Verification items for the finished model (mm, model axes). A direction names the side the tool comes from. Give positions to 0.01 mm unless a question says otherwise; leave off trailing zeros. Order: outer loops, then holes, each group sorted by start corner. A loop starts at its lowest first (then second) coordinate and runs counter-clockwise, first axis right, second up. Notation, with made-up numbers: (13.25, 89) - (67.25, 89) arc R13 cw to (67.25, 99) - close; hole circle Ø8 at (64.25, 20.5). An arc over 180 degrees is marked (long way). Answer as a JSON object with one key per item and string values. Group by question number.
(1) Section check C-C (z = -22). Record the boundary of the cut face in (x, y).
(2) Section check A-A (x = -1.5). Count the separate pieces of the cut face and the enclosed holes in it, then the cut area to 3 significant figures.
(3) Depth check by flat-ended pin: pin 1 Ø1.9 at (x, z) = (-21.5, -22) entering from +Y; pin 2 Ø0.6 at (x, y) = (-15, 6) entering from -Z. Enter the tip coordinate at first touch or a pass-through.
(4) Section check B-B (z = -7.75). Record the boundary of the cut face in (x, y).
(5) Access from +Z, -Z, +X, -X, +Y, -Y to the whole of each face (thin tool, end or side, straight path). Record for faces 1 (the face through (-11, 6.5, -2)), 2 (the face through (-11, 4, -20.5)), 3 (the face through (-11, 5, -17.5)).
(6) Thickness scan on line 1 (Z direction, x = -1.5, y = 1.65); line 2 (X direction, y = 1, z = -22); line 3 (Y direction, x = -5.5, z = -3.5). Record the ranges inside material, lowest first.
(7) Mould release check, pull along Z, two halves, no side actions. Record for faces 4 (the face through (-12, 4.5, -10)), 5 (the face through (-12, 6.5, -19)), 6 (the face through (-12, 3.9, -10)), 7 (the face through (-11, 3, 0)): +Z half, -Z half, draft (parallel to the pull), parting line (faces both ways), or undercut.
(8) Section check D-D (x = -13.5). Record the boundary of the cut face in (y, z).
Autodesk Inventor part; units mm, degrees
ref_plane "YZ Plane" through (0, 0, 0) normal (1, 0, 0) x (0, 1, 0)
ref_plane "XZ Plane" through (0, 0, 0) normal (0, 1, 0) x (-1, 0, 0)
ref_plane "XY Plane" through (0, 0, 0) normal (0, 0, 1) x (1, 0, 0)
sketch "Sketch1" plane through (0, 0, 0) normal (0, 1, 0) x (-1, 0, 0)
  line L0 (0, 0) -> (23, 0)
  line L1 (23, 0) -> (23, -3)
  line L2 (23, -3) -> (0, -3)
  line L3 (0, -3) -> (0, 0)
  line L4 (23, -3) -> (0, -3)
  line L5 (0, -3) -> (0, -17.5)
  line L6 (0, -17.5) -> (23, -17.5)
  line L7 (23, -17.5) -> (23, -3)
  line L8 (23, -17.5) -> (0, -17.5)
  line L9 (0, -17.5) -> (0, -20.5)
  line L10 (0, -20.5) -> (23, -20.5)
  line L11 (23, -20.5) -> (23, -17.5)
  dimension "d0" = 23
  dimension "d1" = 3
  dimension "d2" = 14.5
  dimension "d3" = 3
extrude "Extrusion1" add sketch "Sketch1" along normal blind 5 contours L0 L1 L2 L3 | L6 L11 L10 L9
sketch "Sketch2" plane through (0, 0, -3) normal (0, 0, -1) x (-1, 0, 0)
  line L0 (0, 0) -> (0, 5)
  line L1 (23, 0) -> (23, 5)
  line L2 (0, 1.8) -> (23, 1.8)
  line L3 (23, 1.8) -> (23, 1)
  line L4 (23, 1) -> (0, 1)
  line L5 (0, 1) -> (0, 1.8)
  line L6 (0, 0) -> (23, 0)
  point P0 (0, 1)
  dimension "d6" = 0.8
  dimension "d7" = 1
extrude "Extrusion2" add sketch "Sketch2" along normal up to surface (14.5 mm away) contours L0 L2 L1 L4
sketch "Sketch3" plane through (-23, 5, -17.5) normal (0, 0, 1) x (1, 0, 0)
  line L0 (0, -5) -> (0, 0)
  line L1 (23, -5) -> (23, 0)
  line L2 (0, -1.9) -> (23, -1.9)
  line L3 (23, -1.9) -> (23, -2.7)
  line L4 (23, -2.7) -> (0, -2.7)
  line L5 (0, -2.7) -> (0, -1.9)
  line L6 (0, -3.2) -> (23, -3.2)
  point P0 (0, -2.7)
  dimension "d10" = 0.8
  dimension "d11" = 0.5
extrude "Extrusion3" add sketch "Sketch3" along normal blind 0.7 contours L0 L2 L1 L4
sketch "Sketch4" plane through (0, 5, -3) normal (0, 0, -1) x (-1, 0, 0)
  line L0 (0, -2.7) -> (0, -1.9)
  line L1 (0, -1.9) -> (23, -1.9)
  line L2 (23, -1.9) -> (23, -2.7)
  line L3 (23, -2.7) -> (0, -2.7)
  point P0 (0, -5)
extrude "Extrusion4" add sketch "Sketch4" along normal blind 0.7
sketch "Sketch5" plane through (0, 5, 0) normal (0, 1, 0) x (1, 0, 0)
  line L0 (-23, 0) -> (0, 0)
  line L1 (0, 0) -> (0, 3)
  line L2 (0, 3) -> (-23, 3)
  line L3 (-23, 3) -> (-23, 0)
  line L4 (-23, 17.5) -> (0, 17.5)
  line L5 (0, 17.5) -> (0, 20.5)
  line L6 (0, 20.5) -> (-23, 20.5)
  line L7 (-23, 20.5) -> (-23, 17.5)
extrude "Extrusion5" add sketch "Sketch5" along normal blind 1.5
sketch "Sketch6" plane through (0, 3.1, -3) normal (0, 0, -1) x (-1, 0, 0)
  line L0 (0, 3.4) -> (23, 3.4)
  line L1 (23, 0) -> (23, 3.4)
  line L2 (0, 3.4) -> (23, 3.4)
  line L3 (23, 3.4) -> (23, 2.6)
  line L4 (23, 2.6) -> (0, 2.6)
  line L5 (0, 2.6) -> (0, 3.4)
  point P0 (0, -3.1)
  dimension "d18" = 0.8
extrude "Extrusion6" add sketch "Sketch6" along normal blind 0.7
sketch "Sketch7" plane through (-23, 3.1, -17.5) normal (0, 0, 1) x (1, 0, 0)
  line L0 (23, 2.6) -> (0, 2.6)
  line L1 (0, 2.6) -> (0, 3.4)
  line L2 (0, 3.4) -> (23, 3.4)
  line L3 (23, 3.4) -> (23, 2.6)
  point P0 (23, -3.1)
extrude "Extrusion7" add sketch "Sketch7" along normal blind 0.7
sketch "Sketch8" plane through (-23, 3.1, -17.5) normal (0, 0, 1) x (1, 0, 0)
  line L0 (23, 0) -> (23, 2.6)
  line L1 (0, 0) -> (0, 2.6)
  line L2 (23, 2.1) -> (0, 2.1)
  line L3 (0, 2.1) -> (0, 1.3)
  line L4 (0, 1.3) -> (23, 1.3)
  line L5 (23, 1.3) -> (23, 2.1)
  line L6 (23, 3.4) -> (0, 3.4)
  point P0 (23, -3.1)
  point P1 (0, 2.1)
  dimension "d23" = 0.8
  dimension "d24" = 1.3
extrude "Extrusion8" add sketch "Sketch8" along normal up to surface (14.5 mm away)
sketch "Sketch9" plane through (0, 0, 0) normal (0, -1, 0) x (1, 0, 0)
  line L0 (-23, -17.5) -> (0, -17.5)
  line L1 (-23, -20.5) -> (-23, -17.5)
  line L2 (0, -20.5) -> (-23, -20.5)
  line L3 (0, -17.5) -> (0, -20.5)
  line L4 (-23, 0) -> (0, 0)
  line L5 (-23, -3) -> (-23, 0)
  line L6 (0, -3) -> (-23, -3)
  line L7 (0, 0) -> (0, -3)
extrude "Extrusion9" cut sketch "Sketch9" against normal blind 0.3
sketch "Sketch10" plane through (0, 6.5, -20.5) normal (0, 0, -1) x (-1, 0, 0)
  line L0 (23, -6.2) -> (0, -6.2)
  line L1 (0, -6.2) -> (3, -6.2)
  line L2 (3, -6.2) -> (3, -4.2)
  line L3 (3, -4.2) -> (0, -4.2)
  line L4 (0, -4.2) -> (0, -6.2)
  point P0 (0, -6.5)
  dimension "d29" = 3
  dimension "d30" = 2
extrude "Extrusion10" add sketch "Sketch10" along normal blind 3
sketch "Sketch11" plane through (0, 6.5, -20.5) normal (0, 0, -1) x (-1, 0, 0)
  line L0 (23, -6.2) -> (0, -6.2)
  line L1 (23, -6.2) -> (20, -6.2)
  line L2 (20, -6.2) -> (20, -4.2)
  line L3 (20, -4.2) -> (23, -4.2)
  line L4 (23, -4.2) -> (23, -6.2)
  point P0 (0, -6.5)
  dimension "d33" = 3
  dimension "d34" = 2
extrude "Extrusion11" add sketch "Sketch11" along normal blind 3
sketch "Sketch12" plane through (-3, 2.3, -20.5) normal (0, 1, 0) x (1, 0, 0)
  circle A0 centre (1.5, 1.5) radius 1.05
  line L0 (3, 0) -> (3, 3)
  line L1 (0, 3) -> (3, 3)
  circle A1 centre (-18.5, 1.5) radius 1.05
  line L2 (-17, 0) -> (-17, 3)
  line L3 (-20, 3) -> (-17, 3)
  point P0 (3, -20.5)
  point P1 (1.5, 3)
  point P2 (-17, 1.5)
  point P3 (-18.5, 3)
  dimension "d37" = 2.1
  dimension "d38" = 1.5
  dimension "d39" = 1.5
  dimension "d40" = 2.1
  dimension "d41" = 1.5
  dimension "d42" = 1.5
extrude "Extrusion12" cut sketch "Sketch12" against normal blind 2
sketch "Sketch13" plane through (-20, 0.3, -20.5) normal (1, 0, 0) x (0, 0, -1)
  line L0 (-3, 4.1) -> (-17.5, 4.1)
  line L1 (-3, 2.8) -> (-3, 4.1)
  line L2 (-3, 2.8) -> (-3.7, 2.8)
  line L3 (-3.7, 2) -> (-3.7, 2.8)
  line L4 (-3, 2) -> (-3.7, 2)
  line L5 (-3, 1.5) -> (-3, 2)
  line L6 (-17.5, 1.5) -> (-3, 1.5)
  line L7 (-17.5, 1.5) -> (-17.5, 2)
  line L8 (-17.5, 2) -> (-16.8, 2)
  line L9 (-16.8, 2.8) -> (-16.8, 2)
  line L10 (-17.5, 2.8) -> (-16.8, 2.8)
  line L11 (-17.5, 2.8) -> (-17.5, 4.1)
  line L12 (-20.5, 0) -> (-17.5, 0)
  line L13 (-17.5, 0) -> (-17.5, 0.7)
  line L14 (-17.5, 0.7) -> (-3, 0.7)
  line L15 (-3, 0) -> (-3, 0.7)
  line L16 (-3, 0) -> (3, 0)
  line L17 (3, 2) -> (3, 0)
  line L18 (0, 2) -> (3, 2)
  line L19 (0, 2) -> (0, 6.2)
  line L20 (0, 6.2) -> (-3.7, 6.2)
  line L21 (-3.7, 5.4) -> (-3.7, 6.2)
  line L22 (-3, 5.4) -> (-3.7, 5.4)
  line L23 (-3, 4.9) -> (-3, 5.4)
  line L24 (-3, 4.9) -> (-17.5, 4.9)
  line L25 (-17.5, 4.9) -> (-17.5, 5.4)
  line L26 (-17.5, 5.4) -> (-16.8, 5.4)
  line L27 (-16.8, 6.2) -> (-16.8, 5.4)
  line L28 (-20.5, 6.2) -> (-16.8, 6.2)
  line L29 (-20.5, 0) -> (-20.5, 6.2)
  line L30 (0, 0) -> (0, 2)
  line L31 (0, 0) -> (3, 0)
  line L32 (3, 2) -> (3, 0)
  line L33 (0, 2) -> (3, 2)
  point P0 (-20.5, -0.3)
extrude "Extrusion13" add sketch "Sketch13" along normal up to surface (17 mm away) contours L30 L18 L17 L16
sketch "Sketch14" plane through (-23, 1, -3) normal (0, -1, 0) x (1, 0, 0)
  line L0 (23, -14.5) -> (0, -14.5)
  line L1 (23, 0) -> (23, -14.5)
  line L2 (0, 0) -> (23, 0)
  line L3 (0, 0) -> (0, -14.5)
  point P0 (23, 3)
extrude "Extrusion14" cut sketch "Sketch14" against normal blind 0.8
sketch "Sketch15" plane through (0, 0.3, 0) normal (0, -1, 0) x (1, 0, 0)
  point P0 (0, 0)
sketch "Sketch16" plane through (0, 0.3, 0) normal (0, -1, 0) x (1, 0, 0)
  circle A0 centre (-21.5, -22) radius 1.05
  circle A1 centre (-1.5, -22) radius 1.05
  line L0 (0, -17.5) -> (0, -23.5)
  line L1 (-23, -17.5) -> (0, -17.5)
  line L2 (-23, -23.5) -> (-23, -17.5)
  line L3 (0, -23.5) -> (-23, -23.5)
  line L4 (-23, -3) -> (0, -3)
  line L5 (-23, -17.5) -> (-23, -3)
  line L6 (0, -17.5) -> (-23, -17.5)
  line L7 (0, -17.5) -> (0, -3)
  point P0 (0, 0)
extrude "Extrusion15" add sketch "Sketch16" against normal blind 0.6 contours L1 L5 L4 L7
sketch "Sketch17" plane through (-23, 4.4, -17.5) normal (0, -1, 0) x (1, 0, 0)
  line L0 (0, 14.5) -> (23, 14.5)
  line L1 (0, 0) -> (0, 14.5)
  line L2 (23, 0) -> (0, 0)
  line L3 (23, 0) -> (23, 14.5)
  point P0 (23, 17.5)
extrude "Extrusion16" add sketch "Sketch17" along normal blind 0.5
sketch "Sketch18" plane through (-23, 5.2, -17.5) normal (0, 1, 0) x (1, 0, 0)
  line L0 (23, -14.5) -> (0, -14.5)
  line L1 (23, 0) -> (23, -14.5)
  line L2 (0, 0) -> (23, 0)
  line L3 (0, 0) -> (0, -14.5)
  point P0 (23, -17.5)
extrude "Extrusion17" cut sketch "Sketch18" against normal blind 0.7
properties part number "drvholder" material "Tworzywo sztuczne PET"
Solutions:
{
 "1": {"outline": "(-23, 0.3) - (-22.55, 0.3) - (-22.55, 2.3) - (-23, 2.3) - close; (-20.45, 0.3) - (-2.55, 0.3) - (-2.55, 2.3) - (-20.45, 2.3) - close; (-0.45, 0.3) - (0, 0.3) - (0, 2.3) - (-0.45, 2.3) - close"},
 "2": {"separate pieces": "2", "enclosed holes": "1", "area": "58.6 mm2"},
 "3": {"pin 1": "passes through", "pin 2": "stops at z = -20.5"},
 "4": {"outline": "(-23, 0.3) - (0, 0.3) - (0, 0.9) - (-23, 0.9) - close; (-23, 3.9) - (0, 3.9) - (0, 4.5) - (-23, 4.5) - close"},
 "5": {"face 1": "+Z, -Z, +X, -X, +Y", "face 2": "-Z, +X, -X, +Y", "face 3": "+X, -X"},
 "6": {"line 1": "z = -23.5 to -23.05, -20.95 to -17.5, -3 to 0", "line 2": "x = -23 to -22.55, -20.45 to -2.55, -0.45 to 0", "line 3": "y = 0.3 to 0.9, 2.3 to 3.1, 3.9 to 4.5, 5.7 to 6.5"},
 "7": {"face 4": "undercut", "face 5": "draft", "face 6": "undercut", "face 7": "+Z half"},
 "8": {"outline": "(0.3, -23.5) - (2.3, -23.5) - (2.3, -20.5) - (6.5, -20.5) - (6.5, -16.8) - (5.7, -16.8) - (5.7, -17.5) - (4.5, -17.5) - (4.5, -3) - (5.7, -3) - (5.7, -3.7) - (6.5, -3.7) - (6.5, 0) - (0.3, 0) - close; hole (0.9, -17.5) - (2.3, -17.5) - (2.3, -16.8) - (3.1, -16.8) - (3.1, -17.5) - (3.9, -17.5) - (3.9, -3) - (3.1, -3) - (3.1, -3.7) - (2.3, -3.7) - (2.3, -3) - (0.9, -3) - close"}
}
